Verification items for this drawing (mm, ordinates from the low corner). Give positions to 0.01 mm unless a question says otherwise; leave off trailing zeros. Loops run counter-clockwise (first coordinate to the right, second up) from the corner with the lowest first, then second, coordinate; pieces in that order, holes last. Notation, with made-up numbers: M -26,48 L 29,48 A21 cw 29,66 Z; hole C 45,63 d4. An arc over 180 degrees is marked long. Answer in a Markdown table with one row per item.
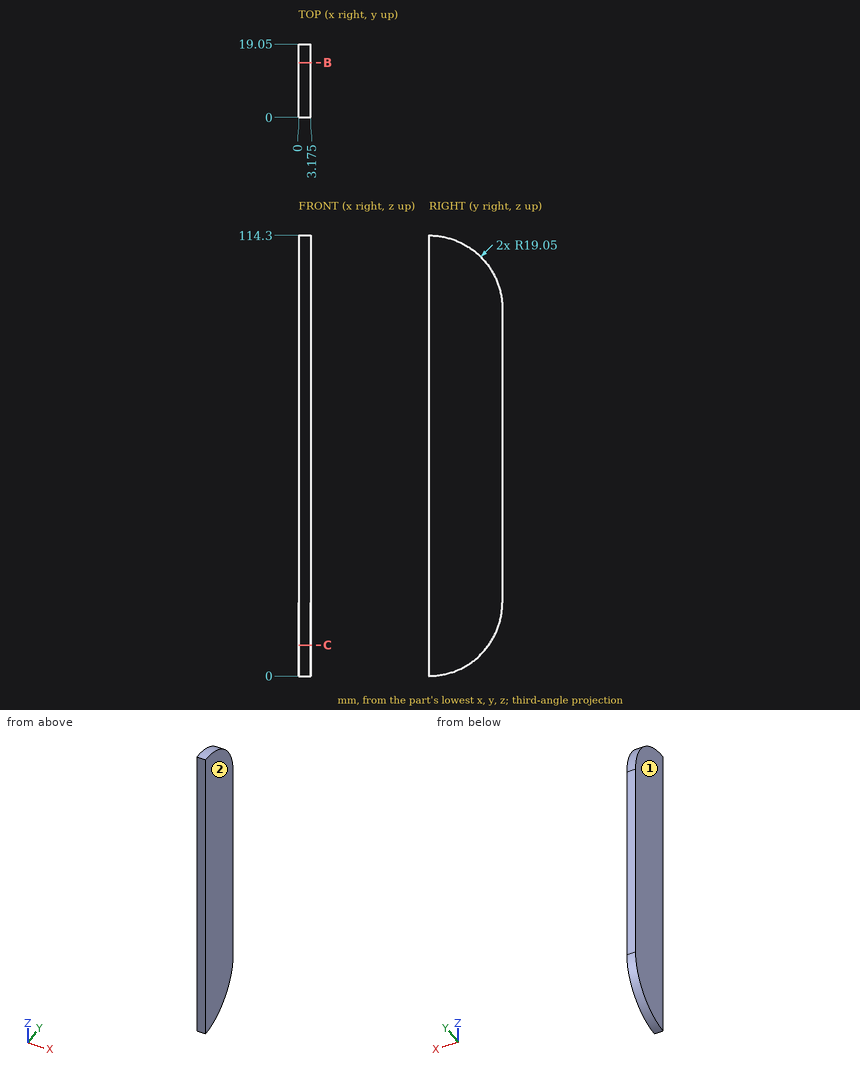
Item 1: Scan lines: L1, parallel to Z at x = 2.4, y = 6.5; L2, parallel to Z at x = 2.75, y = 7; L3, parallel to Y at x = 0.9, z = 107.5. Record each from-to range of solid material in increasing order. Write a range as [from, to].
Reported:
| item | result |
|---|---|
| L1 | z = [1.14, 113.16] |
| L2 | z = [1.33, 112.97] |
| L3 | y = [0, 14.59] |
Item 2: Go/stop test with flat-tipped pins: pin 1 (1.5 mm diameter, centred on x = 1.5, y = 7, fed in from +Z); pin 2 (1 mm diameter, centred on x = 1, y = 15, fed in from -Z) (1 decimal). Record where each tip stops, or that it passes through.
Reported:
| item | result |
|---|---|
| pin 1 | stops at z = 113.25 |
| pin 2 | stops at z = 6.7 |
Item 3: Sectioned sample at C-C (z = 8). Record the cut outline in (x, y) (3 decimals).
Reported:
| item | result |
|---|---|
| outline | M 0,0 L 3.175,0 L 3.175,15.518 L 0,15.518 Z |
Item 4: Sectioned sample at B-B (y = 14.25). Record the cut outline in (x, z) (3 decimals).
Reported:
| item | result |
|---|---|
| outline | M 0,6.407 L 3.175,6.407 L 3.175,107.893 L 0,107.893 Z |
Item 5: Release check for a two-part mould opening along X. For the marked faces 1 and 2 record: released by +X, released by -X, zero draft, split by the parting line, or undercut.
Reported:
| item | result |
|---|---|
| face 1 | released by -X |
| face 2 | released by +X |
